```python
from build123d import *

# Parameters (mm, degrees)
SKETCH_1_W          = 4.5
SKETCH_1_H          = 6
EXTRUDE_1_DEPTH     = 2
SKETCH_2_W          = 19.5
SKETCH_2_H          = 6.5
EXTRUDE_2_DEPTH     = 4.2
SKETCH_4_W          = 10
SKETCH_4_H          = 2.1
EXTRUDE_3_DEPTH     = 4.2
SKETCH_5_W          = 24
SKETCH_5_H          = 3.6
CUT_EXTRUDE_1_DEPTH = 2.95
SKETCH_3_W          = 4.5
SKETCH_3_H          = 3.6
EXTRUDE_4_DEPTH     = 1.5
SKETCH_7_W          = 5.2
SKETCH_7_H          = 3.8
EXTRUDE_5_DEPTH     = 2
CUT_EXTRUDE_2_REACH = 29.339
SKETCH_9_W          = 0.4
SKETCH_9_H          = 5
CUT_EXTRUDE_3_DEPTH = 2.2
FILLET_1_R          = 2.5
CHAMFER_1_SIZE      = 2
SKETCH_10_W         = 9.2
SKETCH_10_H         = 2.5
EXTRUDE_6_DEPTH     = 2.5
SKETCH_11_W         = 17.6
SKETCH_11_H         = 8.6
EXTRUDE_7_DEPTH     = 1.5


with BuildPart() as part:
    # 草图1 → 凸台-拉伸1 (new body)
    with BuildSketch(Plane.XY):
        with Locations((2.25, 3)):
            Rectangle(SKETCH_1_W, SKETCH_1_H)
    extrude(amount=EXTRUDE_1_DEPTH)

    # 草图2 → 凸台-拉伸2 (add)
    with BuildSketch(Plane(origin=(0, 0, 0), x_dir=(-1, 0, 0), z_dir=(0, 0, -1))):
        with Locations((-14.25, 3.25)):
            Rectangle(SKETCH_2_W, SKETCH_2_H)
    extrude(amount=-EXTRUDE_2_DEPTH)

    # 草图4 → 凸台-拉伸3 (add)
    with BuildSketch(Plane(origin=(0, 0, 0), x_dir=(-1, 0, 0), z_dir=(0, 0, -1))):
        with Locations((-19, -1.05)):
            Rectangle(SKETCH_4_W, SKETCH_4_H)
    extrude(amount=-EXTRUDE_3_DEPTH)

    # 草图5 → 切除-拉伸1 (cut)
    with BuildSketch(Plane.XY.offset(4.2)):
        with Locations((12, -0.3)):
            Rectangle(SKETCH_5_W, SKETCH_5_H)
    extrude(amount=-CUT_EXTRUDE_1_DEPTH, mode=Mode.SUBTRACT)

    # 草图3 → 凸台-拉伸4 (add)
    with BuildSketch(Plane(origin=(0, 0, 0), x_dir=(-1, 0, 0), z_dir=(0, 0, -1))):
        with Locations((-21.75, -0.3)):
            Rectangle(SKETCH_3_W, SKETCH_3_H)
    extrude(amount=EXTRUDE_4_DEPTH)

    # 草图7 → 凸台-拉伸5 (add)
    with BuildSketch(Plane(origin=(0, 0, 0), x_dir=(-1, 0, 0), z_dir=(0, 0, -1))):
        with Locations((-7.1, 8.4)):
            Rectangle(SKETCH_7_W, SKETCH_7_H)
    extrude(amount=-EXTRUDE_5_DEPTH)

    # 切除-拉伸2: up to this face of the body (flat: up to its plane)
    cut_extrude_2_end = Plane(part.part.faces().sort_by_distance((2.25, 6, 1))[0])
    # 草图8 → 切除-拉伸2 (cut, up to the picked face)
    with BuildSketch(Plane(origin=(0, 10.3, 0), x_dir=(1, 0, 0), z_dir=(0, 1, 0)), mode=Mode.PRIVATE) as cut_extrude_2_sk1:
        Polygon((4.5, -2), (7.7, 0), (4.5, 0), align=None)
    cut_extrude_2_tool1 = split(extrude(cut_extrude_2_sk1.sketch, amount=-CUT_EXTRUDE_2_REACH, mode=Mode.PRIVATE), bisect_by=cut_extrude_2_end, keep=Keep.BOTH, mode=Mode.PRIVATE)
    add(cut_extrude_2_tool1.solids().sort_by(Axis((5.566667, 10.3, 0.666667), (0, -1, 0)))[0], mode=Mode.SUBTRACT)

    # 草图9 → 切除-拉伸3 (cut)
    with BuildSketch(Plane.XY.offset(4.2)):
        with Locations((4.7, 4)):
            Rectangle(SKETCH_9_W, SKETCH_9_H)
    extrude(amount=-CUT_EXTRUDE_3_DEPTH, mode=Mode.SUBTRACT)

    # 圆角1
    fillet_1_edges = [part.edges().sort_by_distance(p)[0] for p in [
        (24, -2.1, -0.125),
    ]]
    fillet(fillet_1_edges, radius=FILLET_1_R)

    # 倒角1
    chamfer_1_edges = [part.edges().sort_by_distance(p)[0] for p in [
        (24, 6.5, 2.1),
    ]]
    chamfer(chamfer_1_edges, length=CHAMFER_1_SIZE)

    # 草图10 → 凸台-拉伸6 (add)
    with BuildSketch(Plane.XY.offset(4.2)):
        with Locations((12.34, 2.75)):
            Rectangle(SKETCH_10_W, SKETCH_10_H)
    extrude(amount=EXTRUDE_6_DEPTH)

    # 草图11 → 凸台-拉伸7 (add)
    with BuildSketch(Plane.XY.offset(6.7)):
        with Locations((13.7, 2.2)):
            Rectangle(SKETCH_11_W, SKETCH_11_H)
    extrude(amount=EXTRUDE_7_DEPTH)


solid = part.part
```
Check sheet for the modelled part. Datum: model origin and axes. Units: mm. A direction names the side the tool comes from. Give positions to 0.01 mm unless a question says otherwise; leave off trailing zeros. Loops run counter-clockwise (first coordinate to the right, second up) from the corner with the lowest first, then second, coordinate; pieces in that order, holes last. Notation, with made-up numbers: M 83.5,85.5 L 90.5,85.5 A35 cw 90.5,124.5 Z; hole C 2.25,-9.75 d6. An arc over 180 degrees is marked long. Answer in a Markdown table with one row per item.
1) Tool access check on faces 1 (the face through (14, 1.5, 3)), 2 (the face through (22, 1.5, -1)), 3 (the face through (12, 4, 5)). Record the directions out of +Z, -Z, +X, -X, +Y, -Y that give a thin tool (end or side, any length) a straight path to the whole face; none if there is none.
Solutions:
| item | result |
|---|---|
| face 1 | +X, -X, -Y |
| face 2 | -Z, +X, -X, +Y |
| face 3 | +X, -X, +Y |
2) Thickness scan on line 1 (Z direction, x = 6.5, y = 4.25); line 2 (X direction, y = 5.25, z = 7); line 3 (Z direction, x = 1.5, y = 1). Record the ranges inside material, lowest first.
Solutions:
| item | result |
|---|---|
| line 1 | z = 0 to 4.2, 6.7 to 8.2 |
| line 2 | x = 4.9 to 22.5 |
| line 3 | z = 0 to 1.25 |
3) Cross-section at C-C (x = 8.5). Enter the section's corners in (y, z), plus the area to 3 significant figures.
Solutions:
| item | result |
|---|---|
| outline | M -2.1,6.7 L 1.5,6.7 L 1.5,1.25 L 0,1.25 L 0,0 L 10.3,0 L 10.3,2 L 6.5,2 L 6.5,4.2 L 4,4.2 L 4,6.7 L 6.5,6.7 L 6.5,8.2 L -2.1,8.2 Z |
| area | 49.6 mm^2 |
4) Depth check by flat-ended pin: pin 1 (2 mm diameter, centred on x = 20.5, z = 3, fed in from -Y); pin 2 (5 mm diameter, centred on x = 15, z = 1.5, fed in from -Y); pin 3 (1.2 mm diameter, centred on x = 13.5, z = 7.5, fed in from +Y); pin 4 (2 mm diameter, centred on x = 3.5, z = 1, fed in from +Y). Enter the tip coordinate at first touch or a pass-through.
Solutions:
| item | result |
|---|---|
| pin 1 | stops at y = 1.5 |
| pin 2 | stops at y = -2.1 |
| pin 3 | stops at y = 6.5 |
| pin 4 | stops at y = 6 |
5) Cross-section at A-A (y = 0.75). Enter the section's corners in (x, z), plus the area to 4 significant figures.
Solutions:
| item | result |
|---|---|
| outline | M 0,0 L 19.5,0 L 19.5,-1.5 L 24,-1.5 L 24,1.25 L 0,1.25 Z; M 4.9,6.7 L 22.5,6.7 L 22.5,8.2 L 4.9,8.2 Z |
| area | 63.15 mm^2 |
6) Cross-section at D-D (y = 3.25). Enter the section's corners in (x, z).
Solutions:
| item | result |
|---|---|
| outline | M 0,0 L 24,0 L 24,4.2 L 16.94,4.2 L 16.94,6.7 L 22.5,6.7 L 22.5,8.2 L 4.9,8.2 L 4.9,6.7 L 7.74,6.7 L 7.74,4.2 L 4.9,4.2 L 4.9,2 L 0,2 Z |
7) Cross-section at B-B (x = 20.25). Enter the section's corners in (y, z), plus the area to 3 significant figures.
Solutions:
| item | result |
|---|---|
| outline | M -2.1,-1.5 L 1.5,-1.5 L 1.5,0 L 6.5,0 L 6.5,4.2 L 1.5,4.2 L 1.5,1.25 L -2.1,1.25 Z; M -2.1,6.7 L 6.5,6.7 L 6.5,8.2 L -2.1,8.2 Z |
| area | 43.8 mm^2 |
